Part model, mm, in its own coordinate system. A direction names the side the tool comes from. Round coordinates to 2 decimals unless told otherwise and drop trailing zeros. Order: outer loops, then holes, each group sorted by start corner. A loop starts at its lowest first (then second) coordinate and runs counter-clockwise, first axis right, second up. Notation, with made-up numbers: M 33.5,17.25 L 87.5,17.25 A18 cw 87.5,36.25 Z; hole C 35,-38.75 d6. An arc over 180 degrees is marked long. Write each question's results on one line, items separated by ' | '. Start each with the question number.
1. Band-saw the part on A-A, the plane y = 0. List the corners of the cut face in (x, z), then the cut area to 4 significant figures.
2. Probe L1, parallel to Y at x = 0, z = 16; L2, parallel to Z at x = -5, y = 6.5; L3, parallel to Y at x = 0.75, z = 53.5. List the from-to ranges inside material, lowest first. Write a range as [from, to].
3. Drop flat-ended pins along their axis: pin 1 Ø2 at (x, y) = (3.5, -2.5) entering from +Z; pin 2 Ø1.2 at (y, z) = (-1, 67) entering from -X; pin 3 Ø4.5 at (x, z) = (1, 68) entering from +Y. Give the stop position or say it passes through.
4. Which spindle directions (+Z, -Z, +X, -X, +Y, -Y) get a long thin tool onto all of the face, cutting with end or side? Do faces 1 (the face through (3.233, -1.341, 26.138)), 2 (the face through (4, 0, 34.45)), 3 (the face through (0, 2, 67)). Say none if no direction does.
5. Band-saw the part on D-D, the plane y = -4.25. List the corners of the cut face in (x, z).
6. Band-saw the part on C-C, the plane z = 51. List the corners of the cut face in (x, y), then the cut area to 3 significant figures.
```python
from build123d import *

# Parameters (mm, degrees)
CROQUIS1_R              = 3
SALIENTE_EXTRUIR1_DEPTH = 20
CROQUIS2_R              = 3.5
SALIENTE_EXTRUIR2_DEPTH = 12.45
CROQUIS3_R              = 9.5
SALIENTE_EXTRUIR3_DEPTH = 2
CROQUIS4_R              = 3.5
SALIENTE_EXTRUIR4_DEPTH = 4.05
CROQUIS5_R              = 3
SALIENTE_EXTRUIR5_DEPTH = 26
CROQUIS6_W              = 4
CROQUIS6_H              = 4
SALIENTE_EXTRUIR6_DEPTH = 5


with BuildPart() as part:
    # Croquis1 → Saliente-Extruir1 (new body)
    with BuildSketch(Plane.XY):
        Circle(CROQUIS1_R)
    extrude(amount=SALIENTE_EXTRUIR1_DEPTH)

    # Croquis2 → Saliente-Extruir2 (add)
    with BuildSketch(Plane.XY.offset(20)):
        Circle(CROQUIS2_R)
    extrude(amount=SALIENTE_EXTRUIR2_DEPTH)

    # Croquis3 → Saliente-Extruir3 (add)
    with BuildSketch(Plane.XY.offset(32.45)):
        Circle(CROQUIS3_R)
    extrude(amount=SALIENTE_EXTRUIR3_DEPTH)

    # Croquis4 → Saliente-Extruir4 (add)
    with BuildSketch(Plane.XY.offset(34.45)):
        Circle(CROQUIS4_R)
    extrude(amount=SALIENTE_EXTRUIR4_DEPTH)

    # Croquis5 → Saliente-Extruir5 (add)
    with BuildSketch(Plane.XY.offset(38.5)):
        Circle(CROQUIS5_R)
    extrude(amount=SALIENTE_EXTRUIR5_DEPTH)

    # Croquis6 → Saliente-Extruir6 (add)
    with BuildSketch(Plane.XY.offset(64.5)):
        Rectangle(CROQUIS6_W, CROQUIS6_H)
    extrude(amount=SALIENTE_EXTRUIR6_DEPTH)


solid = part.part
```
Solution:
1) outline: M -9.5,32.45 L -3.5,32.45 L -3.5,20 L -3,20 L -3,0 L 3,0 L 3,20 L 3.5,20 L 3.5,32.45 L 9.5,32.45 L 9.5,34.45 L 3.5,34.45 L 3.5,38.5 L 3,38.5 L 3,64.5 L 2,64.5 L 2,69.5 L -2,69.5 L -2,64.5 L -3,64.5 L -3,38.5 L -3.5,38.5 L -3.5,34.45 L -9.5,34.45 Z | area: 449.5 mm^2
2) L1: [-3, 3] | L2: [32.45, 34.45] | L3: [-2.9, 2.9]
3) pin 1: z = 38.5 | pin 2: x = -2 | pin 3: y = 2
4) face 1: -Z | face 2: +Z | face 3: +Z, +X, -X, +Y
5) outline: M -8.5,32.45 L 8.5,32.45 L 8.5,34.45 L -8.5,34.45 Z
6) outline: C 0,0 d6 | area: 28.3 mm^2
